Read the model definition and answer for the solid it produces. Units are mm, in the model's axes. A direction names the side the tool comes from. Give positions to 0.01 mm unless a question says otherwise; leave off trailing zeros. Order: outer loops, then holes, each group sorted by start corner. A loop starts at its lowest first (then second) coordinate and runs counter-clockwise, first axis right, second up. Notation, with made-up numbers: (49, 53) - (53, 53) arc R14 ccw to (53, 79) - close; hole circle Ø4 at (53, 15.5). An arc over 180 degrees is marked (long way). Return JSON: item names as keys, results as strings.
```python
from build123d import *

# Parameters (mm, degrees)
Y_KSEKLIK_EKSTR_ZYON1_DEPTH = 200
Y_KSEKLIK_EKSTR_ZYON3_DEPTH = 200


with BuildPart() as part:
    # Çizim1 → Yükseklik-Ekstrüzyon1 (new body)
    with BuildSketch(Plane.XY):
        Polygon((-5.15760167, 10), (-2.80302277, 5.444963707), (3.391667495, 5.444963707), (5.746246396, 10), (10, 10), (10, 5.45), (5.445076204, 3.095), (5.445076204, -3.095), (10, -5.45), (10, -10), (5.746246396, -10), (3.391667495, -5.444963707), (-2.80302277, -5.444963707), (-5.15760167, -10), (-10, -10), (-10, -5.45), (-5.445076204, -3.095), (-5.445076204, 3.095), (-10, 5.45), (-10, 10), align=None)
    extrude(amount=Y_KSEKLIK_EKSTR_ZYON1_DEPTH)

    # Çizim4 → Yükseklik-Ekstrüzyon3 (add)
    with BuildSketch(Plane.XY.offset(200)):
        Polygon((-5.15760167, 10), (-3.54995598, 10), (-3.54995598, 9.705121592), (-5.005173801, 9.705121592), align=None)
        Polygon((10, 3.84), (9.71, 3.84), (9.71, 5.300063353), (10, 5.45), align=None)
        Polygon((5.593818526, 9.705121592), (5.746246396, 10), (4.138600705, 10), (4.138600705, 9.705121592), align=None)
        Polygon((5.746246396, -10), (4.138600705, -10), (4.138600705, -9.705121592), (5.593818526, -9.705121592), align=None)
        Polygon((-5.005173801, -9.705121592), (-5.15760167, -10), (-3.54995598, -10), (-3.54995598, -9.705121592), align=None)
        Polygon((-10, 5.45), (-10, 3.84), (-9.71, 3.84), (-9.71, 5.300063353), align=None)
        Polygon((9.71, -5.300063353), (10, -5.45), (10, -3.84), (9.71, -3.84), align=None)
        Polygon((-9.71, -5.300063353), (-10, -5.45), (-10, -3.84), (-9.71, -3.84), align=None)
    extrude(amount=-Y_KSEKLIK_EKSTR_ZYON3_DEPTH)


solid = part.part
```
Q1. A cutting plane is placed at B-B (y = 7.25). Write down the section's boundary in (x, z).
Values:
{"outline": "(-10, 0) - (-3.74, 0) - (-3.74, 200) - (-10, 200) - close; (4.32, 0) - (10, 0) - (10, 200) - (4.32, 200) - close"}
Q2. Consider L1, parallel to Y at x = 5, z = 10; L2, parallel to X at y = -5, z = 93; L3, parallel to X at y = -2, z = 86. Determine where each line is inside the solid, lowest interval first.
Values:
{"L1": "y = -10 to -9.71, -8.56 to 8.56, 9.71 to 10", "L2": "x = -10 to -9.71, -9.13 to 9.13, 9.71 to 10", "L3": "x = -5.45 to 5.45"}
Q3. A cutting plane is placed at A-A (x = 7.25). Write down the section's boundary in (y, z).
Values:
{"outline": "(-10, 0) - (-4.03, 0) - (-4.03, 200) - (-10, 200) - close; (4.03, 0) - (10, 0) - (10, 200) - (4.03, 200) - close"}
Q4. Determine the mould class of faces 4 (the flat face through (0, 0, 0)), 5 (the flat face through (5.445, 0, 99)), 6 (the flat face through (-3.89, -7.55, 98.6)) for opening direction X: released by +X, released by -X, zero draft, split by the parting line, or undercut.
Values:
{"face 4": "zero draft", "face 5": "released by +X", "face 6": "undercut"}
Q5. Given pin 1 (5 mm diameter, centred on y = -0.5, z = 127.5, fed in from -X); pin 2 (6 mm diameter, centred on x = 6.5, y = -2.5, fed in from +Z); pin 3 (1.9 mm diameter, centred on y = -1, z = 126.5, fed in from +X); pin 4 (5 mm diameter, centred on x = -0.5, z = 127, fed in from +Y), each flat-ended and moving along its own axis, determine where each tip first touches the part or whether it passes through.
Values:
{"pin 1": "stops at x = -5.45", "pin 2": "stops at z = 200", "pin 3": "stops at x = 5.45", "pin 4": "stops at y = 5.83"}
Q6. For faces 1 (the flat face through (-10, 7, 99)), 2 (the flat face through (0, 5.445, 99)), 3 (the flat face through (-5.445, 0, 99)), determine the directions among +Z, -Z, +X, -X, +Y, -Y from which every point of the face is accessible in a straight line to the end or side of a thin tool.
Values:
{"face 1": "+Z, -Z, -X, +Y, -Y", "face 2": "+Z, -Z, +Y", "face 3": "+Z, -Z, -X"}
